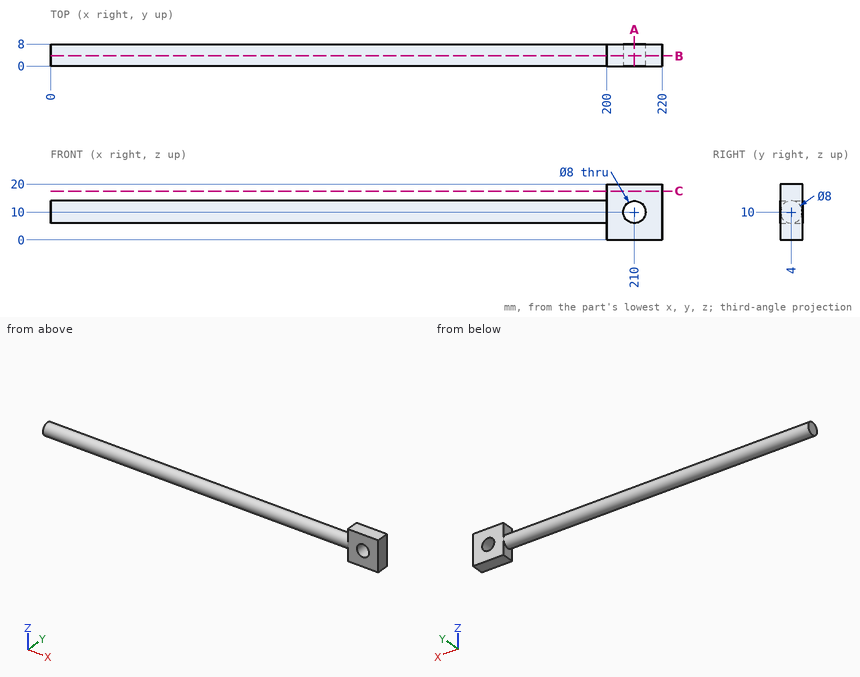
Check sheet for the drawn part. Datum: minimum x, y, z corner. Units: mm. Coordinates: 2 decimals unless noted, no trailing zeros. Write each loop counter-clockwise with the first axis right and the second up, starting at its lowest first coordinate (ties: lowest second). Pieces come first, ordered by that corner, then holes. Notation, with made-up numbers: M 11.25,-8.75 L 24.25,-8.75 A17 cw 24.25,7.25 Z; hole C -23.5,-40 d9. An arc over 180 degrees is marked long. One line per item, written item: value.
Item 1: Section check A-A, the plane x = 210. Record the boundary of the cut face in (y, z), plus the area to 3 significant figures.
Check sheet entries:
outline: M 0,0 L 8,0 L 8,6 L 0,6 Z; M 0,14 L 8,14 L 8,20 L 0,20 Z
area: 96.0 mm^2
Item 2: Scan lines: line 1 along Z through (x, y) = (210, 5.5); line 2 along X through (y, z) = (4.25, 19.25); line 3 along Z through (x, y) = (79.5, 3.75). Record each from-to range of solid material in increasing order.
Check sheet entries:
line 1: z = 0 to 6, 14 to 20
line 2: x = 200 to 220
line 3: z = 6.01 to 13.99
Item 3: Gauge pin test, flat ends, axial feed: pin 1 Ø1 at (x, y) = (44.5, 4) entering from +Z; pin 2 Ø9 at (x, z) = (210, 10) entering from -Y; pin 3 Ø4 at (x, z) = (147.5, 7) entering from -Y; pin 4 Ø4 at (x, y) = (176, 2.5) entering from -Z. Record the tip position at first contact, or that the pin passes through.
Check sheet entries:
pin 1: stops at z = 14
pin 2: stops at y = 0
pin 3: stops at y = 0.13
pin 4: stops at z = 6
Item 4: Section check C-C, the plane z = 17.5. Record the boundary of the cut face in (x, y), plus the area to 3 significant figures.
Check sheet entries:
outline: M 200,0 L 220,0 L 220,8 L 200,8 Z
area: 160 mm^2
Item 5: Section check B-B, the plane y = 3.75. Record the boundary of the cut face in (x, z), plus the area to 3 significant figures.
Check sheet entries:
outline: M 0,6.01 L 200,6.01 L 200,0 L 220,0 L 220,20 L 200,20 L 200,13.99 L 0,13.99 Z; hole C 210,10 d8
area: 1,950 mm^2
